```python
from build123d import *

# Parameters (mm, degrees)
SKETCH2_W                  = 50
SKETCH2_H                  = 30
BOSS_EXTRUDE1_DEPTH        = 25
CUT_EXTRUDE2_DEPTH         = 31
SKETCH7_W                  = 26
SKETCH7_H                  = 21
CUT_EXTRUDE3_DEPTH         = 48
SKETCH8_W                  = 7.000000004
SKETCH8_H                  = 26
CUT_EXTRUDE6_DEPTH         = 3
CUT_EXTRUDE6_DEPTH_BACK    = 10
SKETCH9_W                  = 2
SKETCH9_H                  = 2
BOSS_EXTRUDE2_DEPTH        = 25
BOSS_EXTRUDE2_DEPTH_BACK   = 25
BOSS_EXTRUDE2_2_DEPTH      = 25
BOSS_EXTRUDE2_2_DEPTH_BACK = 25
BOSS_EXTRUDE3_DEPTH        = 30
CUT_EXTRUDE7_DEPTH         = 30
SKETCH13_R                 = 5
BOSS_EXTRUDE4_DEPTH        = 2.5
BOSS_EXTRUDE4_DEPTH_BACK   = 2.5
SKETCH14_R                 = 1.257458731
BOSS_EXTRUDE5_DEPTH        = 2.5
BOSS_EXTRUDE5_DEPTH_BACK   = 7.5
FILLET3_R                  = 2
FILLET4_R                  = 2
FILLET7_R                  = 1
FILLET8_R                  = 1
BOSS_EXTRUDE6_DEPTH        = 5
BOSS_EXTRUDE7_DEPTH        = 5


with BuildPart() as part:
    # Sketch2 → Boss-Extrude1 (new body)
    with BuildSketch(Plane(origin=(0, 0, 0), x_dir=(1, 0, 0), z_dir=(0, 1, 0))):
        Rectangle(SKETCH2_W, SKETCH2_H)
    extrude(amount=BOSS_EXTRUDE1_DEPTH)

    # Sketch3 → Cut-Extrude2 (cut, through all)
    with BuildSketch(Plane.XY.offset(15)):
        with BuildLine():
            Line((-25, 25), (12.5, 16.66666667))
            ThreePointArc((12.5, 16.66666667), (20.568813143, 9.697443192), (25, 0))
            Line((25, 0), (25, 25))
            Line((25, 25), (-25, 25))
        make_face()
    extrude(amount=-CUT_EXTRUDE2_DEPTH, mode=Mode.SUBTRACT)

    # Sketch7 → Cut-Extrude3 (cut)
    with BuildSketch(Plane.ZY.offset(-25)):
        with Locations((0, 12.5)):
            Rectangle(SKETCH7_W, SKETCH7_H)
    extrude(amount=CUT_EXTRUDE3_DEPTH, mode=Mode.SUBTRACT)

    # Sketch8 → Cut-Extrude6 (cut, two sides)
    with BuildSketch(Plane.XZ.offset(-23)) as cut_extrude6_sk:
        with Locations((-19.499999998, 0)):
            Rectangle(SKETCH8_W, SKETCH8_H)
    extrude(amount=CUT_EXTRUDE6_DEPTH, mode=Mode.SUBTRACT)
    extrude(cut_extrude6_sk.sketch, amount=-CUT_EXTRUDE6_DEPTH_BACK, mode=Mode.SUBTRACT)



with BuildPart() as body_2:
    # Sketch9 → Boss-Extrude2 (new body, two sides)
    with BuildSketch(Plane.ZY.offset(-25)) as boss_extrude2_sk:
        with Locations((14, 1)):
            Rectangle(SKETCH9_W, SKETCH9_H)
    extrude(amount=BOSS_EXTRUDE2_DEPTH)
    extrude(boss_extrude2_sk.sketch, amount=-BOSS_EXTRUDE2_DEPTH_BACK)


with BuildPart() as body_3:
    # Sketch9 → Boss-Extrude2 2 (new body, two sides)
    with BuildSketch(Plane.ZY.offset(-25)) as boss_extrude2_2_sk:
        with Locations((-14, 1)):
            Rectangle(SKETCH9_W, SKETCH9_H)
    extrude(amount=BOSS_EXTRUDE2_2_DEPTH)
    extrude(boss_extrude2_2_sk.sketch, amount=-BOSS_EXTRUDE2_2_DEPTH_BACK)


with BuildPart() as part_1:
    add(part.part)

    add(body_2.part)  # Boss-Extrude3 merges body 2

    add(body_3.part)  # Boss-Extrude3 merges body 3
    # Sketch10 → Boss-Extrude3 (add)
    with BuildSketch(Plane.XY.offset(15)):
        Polygon((-25, 0), (-35.654566136, -0.855106022), (-35.494566136, -2.848695749), (-27.301895797, -2.191174678), (0, 0), align=None)
    extrude(amount=-BOSS_EXTRUDE3_DEPTH)

    # Sketch11 → Cut-Extrude7 (cut)
    with BuildSketch(Plane(origin=(-0.16, 1.993589727, 0), x_dir=(0.996794864, 0.08, 0), z_dir=(-0.08, 0.996794864, 0))):
        Polygon((-24.919871589, -15), (-35.608696868, 0), (-35.608696868, -15), align=None)
        Polygon((-35.608696868, 0), (-24.919871589, 15), (-35.608696868, 15), align=None)
    extrude(amount=-CUT_EXTRUDE7_DEPTH, mode=Mode.SUBTRACT)

    # Sketch13 → Boss-Extrude4 (add, two sides)
    with BuildSketch(Plane(origin=(0, 0, 0), x_dir=(-0.08, 0.996794864, 0), z_dir=(0, 0, 1))) as boss_extrude4_sk:
        with Locations((1, 35.608696868)):
            Circle(SKETCH13_R)
    extrude(amount=BOSS_EXTRUDE4_DEPTH)
    extrude(boss_extrude4_sk.sketch, amount=-BOSS_EXTRUDE4_DEPTH_BACK)

    # Sketch14 → Boss-Extrude5 (add, two sides)
    with BuildSketch(Plane.XY.offset(2.5)) as boss_extrude5_sk:
        with Locations((-35.574566136, -1.851900886)):
            Circle(SKETCH14_R)
    extrude(amount=BOSS_EXTRUDE5_DEPTH)
    extrude(boss_extrude5_sk.sketch, amount=-BOSS_EXTRUDE5_DEPTH_BACK)

    # Fillet3
    fillet3_edges = [part_1.edges().sort_by_distance(p)[0] for p in [
        (-40.558540453, -2.251900886, 2.5),
    ]]
    fillet(fillet3_edges, radius=FILLET3_R)

    # Fillet4
    fillet4_edges = [part_1.edges().sort_by_distance(p)[0] for p in [
        (-40.558540453, -2.251900886, -2.5),
    ]]
    fillet(fillet4_edges, radius=FILLET4_R)

    # Fillet7
    fillet7_edges = [part_1.edges().sort_by_distance(p)[0] for p in [
        (-36.832024866, -1.851900886, 5),
    ]]
    fillet(fillet7_edges, radius=FILLET7_R)

    # Fillet8
    fillet8_edges = [part_1.edges().sort_by_distance(p)[0] for p in [
        (-36.832024866, -1.851900886, -5),
    ]]
    fillet(fillet8_edges, radius=FILLET8_R)

    # Sketch15 → Boss-Extrude6 (add)
    with BuildSketch(Plane.XY.offset(15)):
        Polygon((23.647734322, 0), (18.647734702, -5), (13.647734322, 0), align=None)
    extrude(amount=-BOSS_EXTRUDE6_DEPTH)

    # Sketch16 → Boss-Extrude7 (add)
    with BuildSketch(Plane(origin=(0, 0, -15), x_dir=(-1, 0, 0), z_dir=(0, 0, -1))):
        Polygon((-23.647734322, 0), (-18.647734702, -5), (-13.647734322, 0), align=None)
    extrude(amount=-BOSS_EXTRUDE7_DEPTH)


solid = part_1.part
```
Check sheet for the modelled part. Datum: model origin and axes. Units: mm. A direction names the side the tool comes from. Coordinates: 2 decimals unless noted, no trailing zeros. Order: outer loops, then holes, each group sorted by start corner. A loop starts at its lowest first (then second) coordinate and runs counter-clockwise, first axis right, second up. Notation, with made-up numbers: M 75,-16.5 L 116,-16.5 A33 cw 116,19.5 Z; hole C 16,20 d1. An arc over 180 degrees is marked long. One line per question, with ' | ' between items. Start each with the question number.
Item 1: Sectioned sample at D-D on z = -6. Record the cut outline in (x, y), and give its area (3 significant figures).
Item 2: Sectioned sample at C-C on x = 6.5. Record the cut outline in (y, z), and give its area (3 significant figures).
Item 3: Material ranges on line 1 (Z direction, x = -2.5, y = 15); line 2 (X direction, y = 2.5, z = -8.5); line 3 (Y direction, x = 7.5, z = 12.5), recorded low to high.
Item 4: Access from +Z, -Z, +X, -X, +Y, -Y to the whole of each face (thin tool, end or side, straight path). Record for faces 5 (the flat face through (19, -2, -10)), 6 (the flat face through (-4, 11, 13)), 7 (the flat face through (19, 0, 0)).
Item 5: Gauge pin test, flat ends, axial feed: P1, Ø11.5, axis at y = 16.5, z = -0.5, coming from the +X side; P2, Ø8, axis at y = 19, z = 11.5, coming from the +X side; P3, Ø4.5, axis at x = -34.5, y = -1, coming from the -Z side; P4, Ø5, axis at x = 5.5, y = -3.5, coming from the -Z side. Record the tip position at first contact, or that the pin passes through.
Item 6: Mould release check, pull along X, two halves, no side actions. Record for faces 1 (the flat face through (50, 1, -14)), 2 (the flat face through (-29.298, -1.334, 8.838)), 3 (the flat face through (-28.391, -0.272, 0.21)), 4 (the flat face through (19, -2, 10)): pulls with the +X half, pulls with the -X half, needs draft (parallel to the pull), parting line crosses it, or undercut.
Item 7: Sectioned sample at B-B on y = 22. Record the cut outline in (x, z), and give its area (3 significant figures).
Item 8: Sectioned sample at A-A on x = 43.5. Record the cut outline in (y, z), and give its area (3 significant figures).
Answer below:
1) outline: M -31.39,-0.51 L -31.23,-2.51 L 0,0 L 25,0 A25 ccw 24.48,2 L -23,2 L -23,24.56 L -25,25 L -25,0 Z | area: 183 mm^2
2) outline: M 0,-15 L 18,-15 L 18,-13 L 2,-13 L 2,13 L 18,13 L 18,15 L 0,15 Z | area: 124 mm^2
3) line 1: z = -15 to -13, 13 to 15 | line 2: x = -25 to -23 | line 3: y = 0 to 2
4) face 5: +X, -Y | face 6: +X, +Y | face 7: -Y
5) P1: stops at x = -23 | P2: stops at x = 14.74 | P3: stops at z = -5 | P4: passes through
6) face 1: pulls with the +X half | face 2: undercut | face 3: undercut | face 4: needs draft
7) outline: M -25,-15 L -11.5,-15 L -11.5,-13 L -23,-13 L -23,13 L -11.5,13 L -11.5,15 L -25,15 Z | area: 106 mm^2
8) outline: M 0,-15 L 2,-15 L 2,-13 L 0,-13 Z; M 0,13 L 2,13 L 2,15 L 0,15 Z | area: 8.00 mm^2
